The model under review builds one solid part; all positions refer to its coordinate system, in mm. Round coordinates to 2 decimals unless told otherwise and drop trailing zeros. Write each loop counter-clockwise with the first axis right and the second up, starting at its lowest first coordinate (ties: lowest second). Pieces come first, ordered by that corner, then holes. Notation, with made-up numbers: (53, 11.5) - (107, 11.5) arc R22 cw to (107, 49.5) - close; hole circle Ø8 at (-23.75, 25.25). An arc over 180 degrees is marked (long way). Write each question's results on one line, items separated by ' | '.
```python
from build123d import *

# Parameters (mm, degrees)
F0_R     = 20
F2_W     = 40
F2_H     = 40
F4_T     = 1.6
F5_DEPTH = 10


# Not quite as in the source:
# - a shell that OpenCascade refuses in one call is made with other operations: the cavity is built on its own and cut out


with BuildPart() as f3:
    # F0 (on Top) → F3 section 0
    with BuildSketch(Plane.XY):
        Circle(F0_R)
    # F2 (on offset) → F3 section 1
    with BuildSketch(Plane.XY.offset(40)):
        Rectangle(F2_W, F2_H)
    loft()

    # F4: shell of thickness 1.6, made by hand


with BuildPart() as f4_core1:
    # F4_t2: copy of F3
    add(f3.part)

    # the walls: a layer under each face that stays
    f4_faces = [f4_core1.faces().sort_by_distance(p)[0] for p in [
        (19.2387953231, 8.8268343228, 20),
        (0, 19.9999999992, 20),
        (-19.9999999992, 0, 20),
        (0, -19.9999999992, 20),
        (19.2387953231, -8.8268343228, 20),
        (0, 0, 0),
    ]]
    thicken(f4_faces, amount=-F4_T, mode=Mode.SUBTRACT)


with BuildPart() as f3_1:
    add(f3.part)

    # what is left inside the walls is the cavity
    f4_cavity = [f4_core1.part.solids().sort_by_distance(p)[0] for p in [
        (3.677504, 7.355008, 39.984),
    ]]
    add(f4_cavity, mode=Mode.SUBTRACT)

    # F0 (on Top) → F5 (join)
    with BuildSketch(Plane.XY):
        Circle(F0_R)
    extrude(amount=-F5_DEPTH)


solid = f3_1.part
```
Q1. The part is to be moulded in two halves that separate along Y. For faces 1 (the cylindrical face through (-4.336, -19.524, -4.93)), 2 (the flat face through (0, 0, 1.6)), 3 (the flat face through (19, 2, 40)), say which applies: released by +Y, released by -Y, zero draft, split by the parting line, or undercut.
Evaluation:
face 1: split by the parting line | face 2: undercut | face 3: zero draft
Q2. We need section A-A (z = -2.5). State the section outline as (x, y) points.
Evaluation:
outline: circle Ø40 at (0, 0)
Q3. For probe 1 along Y at (x, z) = (0.5, 33); probe 2 along X at (y, z) = (-2, 36); probe 3 along Z at (x, y) = (9, -11.5), list the stretches that pass through material, from the lowest coordinate up.
Evaluation:
probe 1: y = -20 to -18.4, 18.4 to 20 | probe 2: x = -19.99 to -18.39, 18.39 to 19.99 | probe 3: z = -10 to 1.6
Q4. Insertion check: P1, Ø18.5, axis at x = 1, y = -4.5, coming from the +Z side; P2, Ø10, axis at y = 12, z = 21, coming from the +X side; P3, Ø5, axis at y = 14, z = 10.5, coming from the -X side. Each pin has a flat end and moves straight along its axis. Give the tip position at first contact, or say it passes through.
Evaluation:
P1: stops at z = 1.6 | P2: stops at x = 19.57 | P3: stops at x = -17.82
